from build123d import *

# Parameters (mm, degrees)
BOSS_EXTRUDE1_DEPTH = 8


with BuildPart() as part:
    # Sketch1 → Boss-Extrude1 (new body)
    with BuildSketch(Plane.XY):
        Polygon((-178.4, 53), (-150.2, 83.5), (5, 83.5), (5, -3), (-153.2, -3), (-178.4, 20), align=None)
        Polygon((-150.2, 72), (-120.35, 72), (-120.35, 80.5), (-113.85, 80.5), (-113.85, 72), (-36.35, 72), (-36.35, 80.5), (-29.85, 80.5), (-29.85, 72), (0, 72), (0, 40.5), (2, 40.5), (2, 30.5), (0, 30.5), (0, 0), (-150.2, 0), (-150.2, 23), (-175.4, 23), (-175.4, 50), (-150.2, 50), align=None, mode=Mode.SUBTRACT)
    extrude(amount=BOSS_EXTRUDE1_DEPTH)


solid = part.part
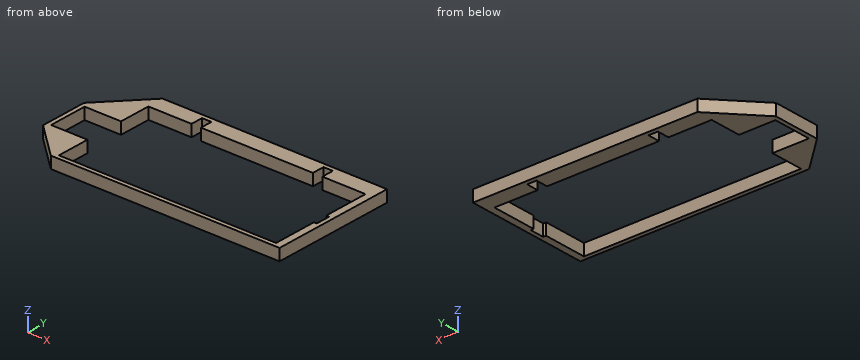
CAD build for the part. Positions are in the model's coordinates, mm. Round coordinates to 2 decimals unless told otherwise and drop trailing zeros. Order: outer loops, then holes, each group sorted by start corner. A loop starts at its lowest first (then second) coordinate and runs counter-clockwise, first axis right, second up. Notation, with made-up numbers: (5.5, 32) - (34.5, 32) arc R10 ccw to (34.5, 39) - close; hole circle Ø3 at (-23.5, -14). An arc over 180 degrees is marked (long way). Return JSON: item names as keys, results as strings.
(1) Cut at C-C (z = 1.5). Give the cut face in (x, y), then the cut area to 3 significant figures.
Answer key:
{"outline": "(-178.4, 20) - (-153.2, -3) - (5, -3) - (5, 83.5) - (-150.2, 83.5) - (-178.4, 53) - close; hole (-175.4, 23) - (-150.2, 23) - (-150.2, 0) - (0, 0) - (0, 30.5) - (2, 30.5) - (2, 40.5) - (0, 40.5) - (0, 72) - (-29.85, 72) - (-29.85, 80.5) - (-36.35, 80.5) - (-36.35, 72) - (-113.85, 72) - (-113.85, 80.5) - (-120.35, 80.5) - (-120.35, 72) - (-150.2, 72) - (-150.2, 50) - (-175.4, 50) - close", "area": "3,520 mm^2"}
(2) Pin check, flat tips, straight feed: pin 1 Ø2.5 at (x, z) = (-158.5, 3.5) entering from -Y; pin 2 Ø2.5 at (y, z) = (74, 2.5) entering from -X. Stop position of each tip, or through.
Answer key:
{"pin 1": "stops at y = 0.7", "pin 2": "stops at x = -160.14"}
(3) Cut at B-B (x = -88). Give the cut face in (y, z), then the cut area to 3 significant figures.
Answer key:
{"outline": "(-3, 0) - (0, 0) - (0, 8) - (-3, 8) - close; (72, 0) - (83.5, 0) - (83.5, 8) - (72, 8) - close", "area": "116 mm^2"}
(4) Cut at A-A (y = 25). Give the cut face in (x, z), then the cut area to 3 significant figures.
Answer key:
{"outline": "(-178.4, 0) - (-175.4, 0) - (-175.4, 8) - (-178.4, 8) - close; (0, 0) - (5, 0) - (5, 8) - (0, 8) - close", "area": "64.0 mm^2"}
(5) Wall check: probe 1 along Y at (x, z) = (-146, 2.5); probe 2 along Y at (x, z) = (-34.5, 4.75); probe 3 along X at (y, z) = (28, 7.5). Give the ranges that are in metal, low to high. Write a range as from..to.
Answer key:
{"probe 1": "y = -3..0, 72..83.5", "probe 2": "y = -3..0, 80.5..83.5", "probe 3": "x = -178.4..-175.4, 0..5"}
